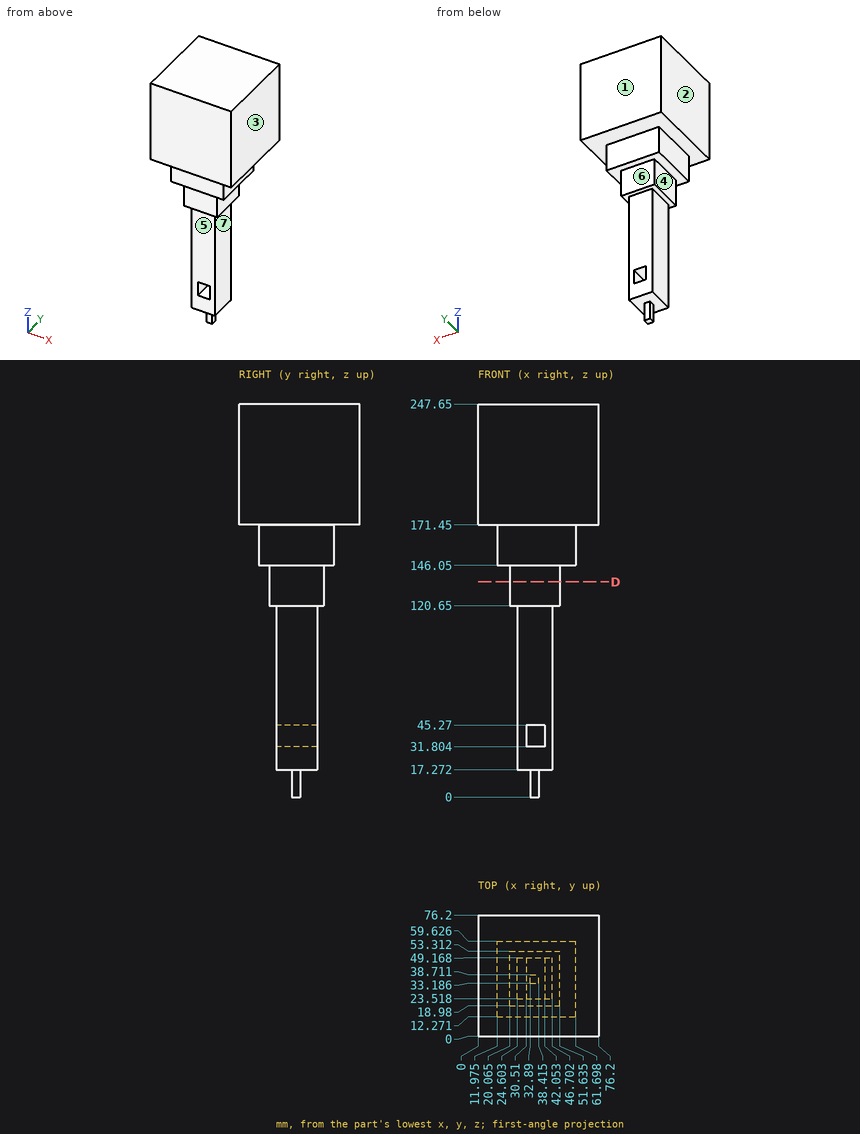
Part print with two shaded views. Sizes in mm from the minimum x, y, z corner. A direction names the side the tool comes from. Coordinates: 2 decimals unless noted, no trailing zeros. Write each loop counter-clockwise with the first axis right and the second up, starting at its lowest first coordinate (ties: lowest second). Pieces come first, ordered by that corner, then holes.
1. Drill centre lines: probe 1 along Z at (x, y) = (31, 33.5); probe 2 along Z at (x, y) = (42.5, 63); probe 3 along Y at (x, z) = (36.5, 137). Where is each one in solid material? Low to high.
Answer block:
probe 1: z = 17.27 to 31.8, 45.27 to 247.65
probe 2: z = 171.45 to 247.65
probe 3: y = 18.98 to 53.31
2. Pull direction X, two halves, no side cores. Call the marked faces 1, 2 and 3: released by +X, released by -X, zero draft, split by the parting line, or undercut.
Answer block:
face 1: zero draft
face 2: released by -X
face 3: released by +X
3. Band-saw the part on D-D, the plane z = 135.5. Give the cut face in (x, y) (1 decimal), and give its area (3 significant figures).
Answer block:
outline: (20.1, 19) - (51.6, 19) - (51.6, 53.3) - (20.1, 53.3) - close
area: 1,080 mm2
4. 3-axis set-ups, long thin cutter, end or side, ignore diameter. For the marked faces 4, 5, 6 and 7: which of +Z, -Z, +X, -X, +Y, -Y reach the whole face in a straight line?
Answer block:
face 4: -Z, -X, +Y, -Y
face 5: -Z, +X, -X, -Y
face 6: -Z, +X, -X, +Y
face 7: -Z, +X, +Y, -Y
5. Drop flat-ended pins along their axis: pin 1 (4.5 mm diameter, centred on x = 35, z = 6, fed in from -Y); pin 2 (6.5 mm diameter, centred on y = 33.5, z = 36, fed in from +X); pin 3 (6 mm diameter, centred on y = 35, z = 6, fed in from +X) (1 decimal). Give the stop position or say it passes through.
Answer block:
pin 1: stops at y = 33.19
pin 2: stops at x = 46.7
pin 3: stops at x = 38.4
